from build123d import *

# Parameters (mm, degrees)
SKETCH1_R                = 50
BOSS_EXTRUDE1_DEPTH      = 50
BOSS_EXTRUDE2_REACH      = 218.16
BOSS_EXTRUDE2_END_RADIUS = 65
SKETCH2_R                = 45


with BuildPart() as part:
    # Sketch1 → Boss-Extrude1 (new, symmetric)
    with BuildSketch(Plane.XY):
        with BuildLine():
            Line((-80, 40), (-80, -40))
            Line((-80, -40), (-22.281665693, -61.061668614))
            ThreePointArc((-22.281665693, -61.061668614), (65, 0), (-22.281665693, 61.061668614))
            Line((-22.281665693, 61.061668614), (-80, 40))
        make_face()
        Circle(SKETCH1_R, mode=Mode.SUBTRACT)
    extrude(amount=BOSS_EXTRUDE1_DEPTH, both=True)

    # Boss-Extrude2: up to this cylinder (the profile starts outside it)
    boss_extrude2_end = Plane(origin=(0, 0, 0), z_dir=(0, 0, -1)) * Cylinder(BOSS_EXTRUDE2_END_RADIUS, 567.32, mode=Mode.PRIVATE)
    # Sketch2 → Boss-Extrude2 (add, up to the surface)
    with BuildSketch(Plane(origin=(120, 0, 0), x_dir=(0, 0, -1), z_dir=(1, 0, 0)), mode=Mode.PRIVATE) as boss_extrude2_sk1:
        Circle(SKETCH2_R)
    boss_extrude2_tool1 = extrude(boss_extrude2_sk1.sketch, amount=-BOSS_EXTRUDE2_REACH, mode=Mode.PRIVATE) - boss_extrude2_end
    add(boss_extrude2_tool1.solids().sort_by_distance((120, 0, 0))[0])

    # Sketch4 → Revolve1 (revolve)
    with BuildSketch(Plane.XY, mode=Mode.PRIVATE) as revolve1_sk:
        Polygon((120, 0), (120, -20), (134, -20), (134, -25), (149, -25), (149, -10.84553833), (158.751026924, -8.628000521), (158.751026924, -5.628000521), (183.498647636, 0), align=None)
    revolve(revolve1_sk.sketch.rotate(Axis((0, 0, 0), (1, 0, 0)), 270), axis=Axis((0, 0, 0), (1, 0, 0)))


solid = part.part
The listing builds one solid part. Answer for the finished solid, in the listing's coordinates (mm). A direction names the side the tool comes from. Round coordinates to 2 decimals unless told otherwise and drop trailing zeros. Write each loop counter-clockwise with the first axis right and the second up, starting at its lowest first coordinate (ties: lowest second). Pieces come first, ordered by that corner, then holes. Notation, with made-up numbers: M 66.5,51.25 L 123.5,51.25 A17 cw 123.5,71.25 Z; hole C 71,52 d4. An arc over 180 degrees is marked long. Write each question's results on one line, items separated by ' | '. Start each with the question number.
Item 1: Which of the six approach directions +Z, -Z, +X, -X, +Y, -Y give full straight-line access (tool end or side, diameter ignored) to faces 5 (the flat face through (-41, 30, 50)), 6 (the cylindrical face through (141.605, -7.509, 23.846)), 7 (the flat face through (134, -17, 11))?
Item 2: Find section A-A on x = 0. Write down the section's boundary in (y, z).
Item 3: Given pin 1 Ø4 at (y, z) = (-42.5, 22.5) entering from +X; pin 2 Ø14 at (y, z) = (0, -2) entering from +X; pin 3 Ø1 at (x, z) = (12, -6) entering from -Y; pin 4 Ø6 at (x, z) = (50.5, 5) entering from -Y, each flat-ended and moving along its own axis, determine where each tip first touches the part or whether it passes through.
Item 4: Find section C-C on y = 17.5. Write down the section's boundary in (x, z).
Item 5: Find section B-B on z = 37. Write down the section's boundary in (x, y), and give its area (3 significant figures).
Item 6: Find section D-D on x = -35.5. Write down the section's boundary in (y, z).
Item 7: Straight lines are drawn through the part: probe 1 along X at (y, z) = (-0.5, -21); probe 2 along Y at (x, z) = (0, 2); probe 3 along X at (y, z) = (1.5, 29). For each, find the intervals that lie inside material, in ascending order.
Item 8: The mould has two halves that part along X. Classify faces 1 (the cylindrical face through (84, -27, 36)), 2 (the conical face through (171.3, 2.71, -0.6)), 3 (the flat face through (-51.5, -50.4, 0.7)), 4 (the cylindrical face through (47.69, 15.02, -0.7)): +X half, -X half, draft (parallel to the pull), parting line (faces both ways), or undercut.
Answer block:
1) face 5: +Z, +X, -X, +Y, -Y | face 6: +X | face 7: none
2) outline: M -65,-50 L -50,-50 L -50,50 L -65,50 Z; M 50,-50 L 65,-50 L 65,50 L 50,50 Z
3) pin 1: stops at x = 50.84 | pin 2: stops at x = 183.5 | pin 3: stops at y = -63.97 | pin 4: stops at y = -44.96
4) outline: M -80,-50 L -46.84,-50 L -46.84,50 L -80,50 Z; M 46.84,-50 L 62.6,-50 L 62.6,-41.46 L 120,-41.46 L 120,-9.68 L 134,-9.68 L 134,-17.85 L 149,-17.85 L 149,17.85 L 134,17.85 L 134,9.68 L 120,9.68 L 120,41.46 L 62.6,41.46 L 62.6,50 L 46.84,50 Z
5) outline: M -80,-40 L -22.28,-61.06 A65 ccw 59.74,-25.61 L 120,-25.61 L 120,25.61 L 59.74,25.61 A65 ccw -22.28,61.06 L -80,40 Z; hole C 0,0 d100 | area: 10,400 mm²
6) outline: M -56.24,-50 L -35.21,-50 L -35.21,50 L -56.24,50 Z; M 35.21,-50 L 56.24,-50 L 56.24,50 L 35.21,50 Z
7) probe 1: x = -80 to -50, 50 to 120, 134 to 149 | probe 2: y = -65 to -50, 50 to 65 | probe 3: x = -80 to -49.98, 49.98 to 120
8) face 1: draft | face 2: +X half | face 3: -X half | face 4: undercut
